Verification items for the finished model (mm, model axes). A direction names the side the tool comes from. Round coordinates to 2 decimals unless told otherwise and drop trailing zeros. Write each loop counter-clockwise with the first axis right and the second up, starting at its lowest first coordinate (ties: lowest second). Pieces come first, ordered by that corner, then holes.
from build123d import *

# Parameters (mm, degrees)
F0_W     = 38.1
F0_H     = 44.45
F1_DEPTH = 76.2
F2_R     = 19.04999
F3_R     = 12.7
F4_DEPTH = 76.201
F5_R     = 1.651
F6_DEPTH = 12.7


# Not quite as in the source:
# - a fillet or chamfer is up to 0.001 mm smaller than in the source, because OpenCascade refuses the exact size


with BuildPart() as f1:
    # F0 (on Front) → F1 (new body)
    with BuildSketch(Plane.XZ):
        with Locations((19.05, 22.225)):
            Rectangle(F0_W, F0_H)
    extrude(amount=F1_DEPTH)

    # F2 (radius 19.05 in the source; OpenCascade refuses exactly that, so slightly less here)
    f2_edges = [f1.edges().sort_by_distance(p)[0] for p in [
        (0, -38.1, 44.45),
        (38.1, -38.1, 44.45),
    ]]
    fillet(f2_edges, radius=F2_R)

    # F3 (on face) → F4 (cut, through all)
    with BuildSketch(Plane.XZ.offset(76.2)):
        with Locations((19.05, 25.4)):
            Circle(F3_R)
    extrude(amount=-F4_DEPTH, mode=Mode.SUBTRACT)

    # F5 (on face) → F6 (cut)
    with BuildSketch(Plane(origin=(0, 0, 0), x_dir=(1, 0, 0), z_dir=(0, 0, -1))):
        with Locations((31.75, 69.85)):
            Circle(F5_R)
        with Locations((6.35, 69.85)):
            Circle(F5_R)
        with Locations((31.75, 6.35)):
            Circle(F5_R)
        with Locations((6.35, 6.35)):
            Circle(F5_R)
    extrude(amount=-F6_DEPTH, mode=Mode.SUBTRACT)


solid = f1.part
Q1. Tool access check on faces 4 (the flat face through (6, -6, 12.7)), 5 (the cylindrical face through (25.877, -38.633, 36.109)). Record the directions out of +Z, -Z, +X, -X, +Y, -Y that give a thin tool (end or side, any length) a straight path to the whole face; none if there is none.
Recorded:
face 4: -Z
face 5: +Y, -Y
Q2. Material ranges on line 1 along X through (y, z) = (-6.35, 9.5); line 2 along Y through (x, z) = (6.35, 9.75); line 3 along Z through (x, y) = (18, -22.5), recorded low to high.
Recorded:
line 1: x = 0 to 4.7, 8 to 30.1, 33.4 to 38.1
line 2: y = -76.2 to -71.5, -68.2 to -8, -4.7 to 0
line 3: z = 0 to 12.74, 38.06 to 44.42
Q3. Depth check by flat-ended pin: P1, Ø12, axis at x = 23, z = 22.5, coming from the -Y side; P2, Ø2.5, axis at x = 31.75, y = -6.35, coming from the -Z side; P3, Ø4.5, axis at x = 31.75, y = -69.85, coming from the +Z side. Enter the tip coordinate at first touch or a pass-through.
Recorded:
P1: passes through
P2: stops at z = 12.7
P3: stops at z = 41.33
Q4. Sectioned sample at C-C (x = 21). Enter the section's corners in (y, z).
Recorded:
outline: (-76.2, 0) - (0, 0) - (0, 12.85) - (-76.2, 12.85) - close; (-76.2, 37.95) - (0, 37.95) - (0, 44.35) - (-76.2, 44.35) - close
Q5. Sectioned sample at B-B (z = 29.5). Enter the section's corners in (x, y), plus the area to 3 significant figures.
Recorded:
outline: (0.45, -76.2) - (7.03, -76.2) - (7.03, 0) - (0.45, 0) - close; (31.07, -76.2) - (37.65, -76.2) - (37.65, 0) - (31.07, 0) - close
area: 1,000 mm2
Q6. Release check for a two-part mould opening along X. For faces 1 (the flat face through (15, -76.2, 13)), 2 (the flat face through (6, -70, 12.7)), 3 (the cylindrical face through (5.43, -38.63, 38.72)) record: released by +X, released by -X, zero draft, split by the parting line, or undercut.
Recorded:
face 1: zero draft
face 2: undercut
face 3: released by -X
